Could you check a few things on this model? Use its own coordinates, in mm. A direction names the side the tool comes from. Coordinates: 2 decimals unless noted, no trailing zeros. Write each loop counter-clockwise with the first axis right and the second up, starting at its lowest first coordinate (ties: lowest second). Pieces come first, ordered by that corner, then holes.
Item 1: If I drill on probe 1 along Y at (x, z) = (-9, 6.75); probe 2 along Y at (x, z) = (0, 21.75); probe 3 along Z at (x, y) = (12, -7), over which ranges is the centre line in solid material (lowest first)?
Item 2: For P1, Ø7, axis at x = 0, y = 0, coming from the +Z side; P2, Ø5.5, axis at x = -0.5, z = 17, coming from the +Y side; P3, Ø7, axis at x = 10.61, y = 10.61, coming from the +Z side; P4, Ø2, axis at x = 2.5, y = 6, coming from the -Z side, each with a flat end and sliding along its axis, tell me the tip position at first contact or that it passes through.
Item 3: Which directions (+Z, -Z, +X, -X, +Y, -Y) give clear straight access to the entire face, cutting with the end or side of a thin tool? Please do faces 4 (the flat face through (6, -3, 28.7)), 5 (the flat face through (-1, 14.6, 11.5)), 6 (the flat face through (6, 0, 19.7)).
Item 4: I want a section at C-C on y = 14.5. Please give me the cut outline in (x, z), then the cut area to 3 significant figures.
Item 5: I want a section at A-A on y = 0. Please give me the cut outline in (x, z), then the cut area to 3 significant figures.
Item 6: I want a section at D-D on x = 0.5. State how many separate pieces and enclosed holes the cut face has, then the cut area to 3 significant figures.
Item 7: I want a section at B-B on z = 6.5. Please give me the cut outline in (x, y) (3 decimals).
Item 8: Thinking about a two-plate mould opening in X: for faces 1 (the flat face through (1.01, 17.4, 11.49)), 2 (the cylindrical face through (-10.886, 12.738, 5.577)), 3 (the flat face through (-4, -7, 29.7)), which applies, +X half, -X half, draft (parallel to the pull), parting line (faces both ways), or undercut?
from build123d import *
from build123d.topology import SkipClean

# Parameters (mm, degrees)
SKETCH1_R           = 20
SKETCH1_R_2         = 4.75
BOSS_EXTRUDE1_DEPTH = 11
SKETCH2_W           = 13.186598354
SKETCH2_H           = 1
SKETCH2_W_2         = 3
SKETCH2_H_2         = 26.426474467
SKETCH2_H_3         = 26.621798467
SKETCH2_W_3         = 40.686040312
SKETCH2_H_4         = 3
CUT_EXTRUDE1_DEPTH  = 31.347981811
SKETCH3_R           = 2.15
CUT_EXTRUDE2_DEPTH  = 28.766886754
SKETCH5_R           = 0.9
BOSS_EXTRUDE2_DEPTH = 18.7
SKETCH13_R          = 0.9
BOSS_EXTRUDE3_DEPTH = 8.7
SKETCH7_W           = 68.268212127
SKETCH7_H           = 3
CUT_EXTRUDE4_DEPTH  = 1
SKETCH10_R          = 4.75
CUT_EXTRUDE6_DEPTH  = 40.141921261
SKETCH11_W          = 9.5
SKETCH11_H          = 3
CUT_EXTRUDE7_DEPTH  = 7
SKETCH12_R          = 6
CUT_EXTRUDE8_DEPTH  = 14.7
CHAMFER2_SIZE       = 1.5
CHAMFER1_SIZE       = 4
CHAMFER1_SIZE2      = 4.76701437
FILLET2_R           = 10
SKETCH14_W          = 5
SKETCH14_H          = 3.3
CUT_EXTRUDE9_DEPTH  = 10
BOSS_EXTRUDE4_DEPTH = 1


with BuildPart() as part:
    # Sketch1 → Boss-Extrude1 (new body)
    with BuildSketch(Plane.XY):
        Circle(SKETCH1_R)
        Circle(SKETCH1_R_2, mode=Mode.SUBTRACT)
    extrude(amount=BOSS_EXTRUDE1_DEPTH)

    # Sketch2 → Cut-Extrude1 (cut, through all)
    with BuildSketch(Plane.XY.offset(11)):
        with Locations((0, 19.5)):
            Rectangle(SKETCH2_W, SKETCH2_H)
        with Locations((-18.5, 2.677583481)):
            Rectangle(SKETCH2_W_2, SKETCH2_H_2)
        with Locations((18.5, -1.585343055)):
            Rectangle(SKETCH2_W_2, SKETCH2_H_3)
        with Locations((1.398669187, -18.5)):
            Rectangle(SKETCH2_W_3, SKETCH2_H_4)
    extrude(amount=-CUT_EXTRUDE1_DEPTH, mode=Mode.SUBTRACT)

    # Sketch3 → Cut-Extrude2 (cut, through all)
    with BuildSketch(Plane.XY.offset(11)):
        with Locations((-10.606601718, -10.606601718)):
            Circle(SKETCH3_R)
        with Locations((-10.606601718, 10.606601718)):
            Circle(SKETCH3_R)
        with Locations((10.606601718, 10.606601718)):
            Circle(SKETCH3_R)
        with Locations((10.606601718, -10.606601718)):
            Circle(SKETCH3_R)
    extrude(amount=-CUT_EXTRUDE2_DEPTH, mode=Mode.SUBTRACT)

    # Sketch5 → Boss-Extrude2 (add)
    with BuildSketch(Plane.XY.offset(11)):
        with BuildLine():
            Line((7.5, -4), (7.5, 4))
            ThreePointArc((7.5, 4), (6.035533906, 7.535533906), (2.5, 9))
            Line((2.5, 9), (-2.5, 9))
            ThreePointArc((-2.5, 9), (-6.035533906, 7.535533906), (-7.5, 4))
            Line((-7.5, 4), (-7.5, -4))
            ThreePointArc((-7.5, -4), (-6.035533906, -7.535533906), (-2.5, -9))
            Line((-2.5, -9), (2.5, -9))
            ThreePointArc((2.5, -9), (6.035533906, -7.535533906), (7.5, -4))
        make_face()
        with Locations(Location((-5.75, 0, 0), (0, 0, 270))):
            Circle(SKETCH5_R, mode=Mode.SUBTRACT)
        with Locations(Location((5.75, 0, 0), (0, 0, 270))):
            Circle(SKETCH5_R, mode=Mode.SUBTRACT)
    extrude(amount=BOSS_EXTRUDE2_DEPTH)

    # Sketch13 → Boss-Extrude3 (add)
    with BuildSketch(Plane.XY.offset(11)):
        with Locations(Location((5.75, 0, 0), (0, 0, 270))):
            Circle(SKETCH13_R)
        with Locations(Location((-5.75, 0, 0), (0, 0, 270))):
            Circle(SKETCH13_R)
    extrude(amount=BOSS_EXTRUDE3_DEPTH)

    # Sketch7 → Cut-Extrude4 (cut)
    with BuildSketch(Plane.XY.offset(29.7)):
        with Locations((-6.527699882, -3.5)):
            Rectangle(SKETCH7_W, SKETCH7_H)
    extrude(amount=-CUT_EXTRUDE4_DEPTH, mode=Mode.SUBTRACT)

    # Sketch10 → Cut-Extrude6 (cut, through all)
    with SkipClean():  # the faces are left unmerged after this step: merging them gives an invalid solid
        with BuildSketch(Plane(origin=(0, 0, 0), x_dir=(-1, 0, 0), z_dir=(0, 0, -1))):
            with Locations(Location((0, 0, 0), (0, 0, 335.09893763))):
                Circle(SKETCH10_R)
        extrude(amount=-CUT_EXTRUDE6_DEPTH, mode=Mode.SUBTRACT)

    # Sketch11 → Cut-Extrude7 (cut)
    with SkipClean():  # the faces are left unmerged after this step: merging them gives an invalid solid
        with BuildSketch(Plane(origin=(0, 9, 0), x_dir=(1, 0, 0), z_dir=(0, 1, 0))):
            with Locations((0, -27.9)):
                Rectangle(SKETCH11_W, SKETCH11_H)
        extrude(amount=-CUT_EXTRUDE7_DEPTH, mode=Mode.SUBTRACT)

    # Sketch12 → Cut-Extrude8 (cut)
    with BuildSketch(Plane(origin=(0, 0, 0), x_dir=(-1, 0, 0), z_dir=(0, 0, -1))):
        Circle(SKETCH12_R)
    extrude(amount=-CUT_EXTRUDE8_DEPTH, mode=Mode.SUBTRACT)

    # Chamfer2
    # the kernel refuses this chamfer: 1.5 mm, written as the material it adds along each edge
    with BuildSketch(Plane(origin=(0, 0, 14.7), x_dir=(-1, 0, 0), z_dir=(0, -1, 0))) as chamfer2_piece_1_section:
        Polygon((6, CHAMFER2_SIZE), (6 - CHAMFER2_SIZE, 0), (6, 0), align=None)
    chamfer2_piece_1 = revolve(axis=Axis((0, 0, 14.7), (0, 0, -1)), mode=Mode.PRIVATE)
    chamfer2_piece_1 = chamfer2_piece_1 - Plane(origin=(0, 0, 14.7), x_dir=(-0.9070362073508065, -0.4210526315731381, 0), z_dir=(0, 0, -1)) * Cylinder(4.75, 24, mode=Mode.PRIVATE)
    add(chamfer2_piece_1)

    # Chamfer1
    chamfer1_edges = [part.edges().sort_by_distance(p)[0] for p in [
        (6, 0, 0),
    ]]
    chamfer1_side = [part.faces().sort_by_distance(p)[0] for p in [
        (16.504823264, 0, 0),
    ]]
    chamfer(chamfer1_edges, length=CHAMFER1_SIZE, length2=CHAMFER1_SIZE2, reference=chamfer1_side[0])

    # Fillet2
    # the kernel refuses this fillet: 10 mm, written as the material it adds along each edge
    with BuildSketch(Plane(origin=(4.75, 2, 29.4), x_dir=(-1, 0, 0), z_dir=(0, 0, -1)), Plane(origin=(-4.75, 2, 19.052989911), x_dir=(1, 0, 0), z_dir=(0, 0, 1))) as fillet2_piece_1:
        with BuildLine():
            CenterArc((10, 2.938804035), FILLET2_R, 180, 17.090413612)
            Line((0, 2.938804035), (-0.2, 2.938804035))
            Line((-0.2, 2.938804035), (-0.2, 0))
            Line((-0.2, 0), (0, -0.2))
            ThreePointArc((0, -0.2), (0.220789008, -0.2), (0.250409575, -0.058776081))
            Line((0.250409575, -0.058776081), (0.441578015, 0))
        make_face()
    extrude(amount=10.347010089)

    # Sketch14 → Cut-Extrude9 (cut)
    with BuildSketch(Plane.XZ.offset(9)):
        with Locations((0, 28.05)):
            Rectangle(SKETCH14_W, SKETCH14_H)
    extrude(amount=-CUT_EXTRUDE9_DEPTH, mode=Mode.SUBTRACT)

    # Sketch15 → Boss-Extrude4 (add)
    with BuildSketch(Plane.XY.offset(11)):
        Polygon((-1, 13.002035862), (1, 13.002035862), (1, 16.164200489), (2, 16.164200489), (0, 18.664200489), (-2, 16.164200489), (-1, 16.164200489), align=None)
    extrude(amount=BOSS_EXTRUDE4_DEPTH)


solid = part.part
Response values:
1. probe 1: y = -17 to -12.04, -9.18 to 9.18, 12.04 to 17.86
1. probe 2: y = -9 to -4.75, 4.75 to 9
1. probe 3: z = 0 to 11
2. P1: passes through
2. P2: stops at y = 9
2. P3: stops at z = 11
2. P4: stops at z = 2.98
3. face 4: +Z, +X, -X
3. face 5: +Z, -X
3. face 6: +Z
4. outline: (-13.77, 0) - (13.77, 0) - (13.77, 11) - (1, 11) - (1, 12) - (-1, 12) - (-1, 11) - (-13.77, 11) - close
4. area: 305 mm2
5. outline: (-17, 0) - (-10, 0) - (-6, 4.77) - (-6, 13.2) - (-4.75, 14.45) - (-4.75, 29.7) - (-4.85, 29.7) - (-4.85, 19.7) - (-6.65, 19.7) - (-6.65, 29.7) - (-7.5, 29.7) - (-7.5, 11) - (-17, 11) - close; (4.75, 14.45) - (6, 13.2) - (6, 4.77) - (10, 0) - (17, 0) - (17, 11) - (7.5, 11) - (7.5, 29.7) - (6.65, 29.7) - (6.65, 19.7) - (4.85, 19.7) - (4.85, 29.7) - (4.75, 29.7) - close
5. area: 283 mm2
6. separate pieces: 3
6. enclosed holes: 0
6. area: 376 mm2
7. outline: (-17, -10.536) arc R20 ccw to (-10.536, -17) - (10.536, -17) arc R20 ccw to (17, -10.536) - (17, 10.536) arc R20 ccw to (6.245, 19) - (-6.245, 19) arc R20 ccw to (-17, 10.536) - close; hole circle Ø4.3 at (-10.607, -10.607); hole circle Ø4.3 at (-10.607, 10.607); hole circle Ø12 at (0, 0); hole circle Ø4.3 at (10.607, -10.607); hole circle Ø4.3 at (10.607, 10.607)
8. face 1: +X half
8. face 2: undercut
8. face 3: draft
